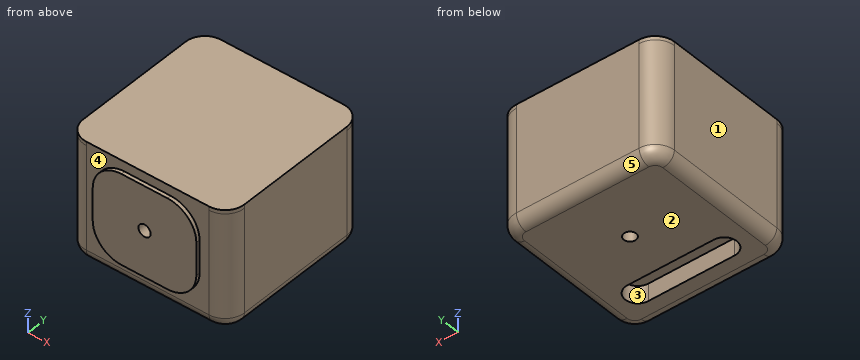
```python
from build123d import *

# Parameters (mm, degrees)
ESQUISSE1_W             = 84
ESQUISSE1_H             = 84
BOSS_EXTRU_1_DEPTH      = 60
CONG_1_R                = 10
CONG_2_R                = 6
BOSS_EXTRU_2_DEPTH      = 2
ESQUISSE5_R             = 3.175
ENL_V_MAT_EXTRU_1_DEPTH = 6
ENL_V_MAT_EXTRU_2_DEPTH = 9
ESQUISSE7_R             = 3.175
ENL_V_MAT_EXTRU_3_DEPTH = 6
BOSS_EXTRU_3_START      = 2
BOSS_EXTRU_3_DEPTH      = 2


with BuildPart() as part:
    # Esquisse1 → Boss.-Extru.1 (new body)
    with BuildSketch(Plane.XY):
        with Locations((12.35180193, 14.109375)):
            Rectangle(ESQUISSE1_W, ESQUISSE1_H)
    extrude(amount=BOSS_EXTRU_1_DEPTH)

    # Congé1
    cong_1_edges = [part.edges().sort_by_distance(p)[0] for p in [
        (-29.64819807, 56.109375, 30),
        (54.35180193, 56.109375, 30),
        (54.35180193, -27.890625, 30),
        (-29.64819807, -27.890625, 30),
    ]]
    fillet(cong_1_edges, radius=CONG_1_R)

    # Congé2
    cong_2_edges = [part.edges().sort_by_distance(p)[0] for p in [
        (12.35180193, -27.890625, 0),
        (-29.64819807, 14.109375, 0),
        (12.35180193, 56.109375, 0),
        (54.35180193, 14.109375, 0),
        (51.422869741, 53.180442812, 0),
        (-26.719265882, 53.180442812, 0),
        (51.422869741, -24.961692812, 0),
        (-26.719265882, -24.961692812, 0),
    ]]
    fillet(cong_2_edges, radius=CONG_2_R)

    # Esquisse2 → Boss.-Extru.2 (add)
    with BuildSketch(Plane.XZ.offset(27.890625)):
        with BuildLine():
            Line((24.35180193, 57), (0.35180193, 57))
            ThreePointArc((0.35180193, 57), (-10.254799788, 52.606601718), (-14.64819807, 42))
            Line((-14.64819807, 42), (-14.64819807, 25))
            ThreePointArc((-14.64819807, 25), (-10.254799788, 14.393398282), (0.35180193, 10))
            Line((0.35180193, 10), (24.35180193, 10))
            ThreePointArc((24.35180193, 10), (34.958403647, 14.393398282), (39.35180193, 25))
            Line((39.35180193, 25), (39.35180193, 42))
            ThreePointArc((39.35180193, 42), (34.958403647, 52.606601718), (24.35180193, 57))
        make_face()
    extrude(amount=BOSS_EXTRU_2_DEPTH)

    # Esquisse5 → Enlèv. mat.-Extru.1 (cut)
    with BuildSketch(Plane.XZ.offset(29.890625)):
        with Locations(Location((12.35180193, 34, 0), (0, 0, 270))):
            Circle(ESQUISSE5_R)
    extrude(amount=-ENL_V_MAT_EXTRU_1_DEPTH, mode=Mode.SUBTRACT)

    # Esquisse6 → Enlèv. mat.-Extru.2 (cut)
    with BuildSketch(Plane(origin=(0, 0, 0), x_dir=(-1, 0, 0), z_dir=(0, 0, -1))):
        with BuildLine():
            Line((-34.85180193, -1.890625), (10.14819807, -1.890625))
            ThreePointArc((10.14819807, -1.890625), (16.64819807, -8.390625), (10.14819807, -14.890625))
            Line((10.14819807, -14.890625), (-34.85180193, -14.890625))
            ThreePointArc((-34.85180193, -14.890625), (-41.35180193, -8.390625), (-34.85180193, -1.890625))
        make_face()
    extrude(amount=-ENL_V_MAT_EXTRU_2_DEPTH, mode=Mode.SUBTRACT)

    # Esquisse7 → Enlèv. mat.-Extru.3 (cut)
    with BuildSketch(Plane(origin=(0, 0, 0), x_dir=(-1, 0, 0), z_dir=(0, 0, -1))):
        with Locations((-14.35180193, 21.109375)):
            Circle(ESQUISSE7_R)
    extrude(amount=-ENL_V_MAT_EXTRU_3_DEPTH, mode=Mode.SUBTRACT)

    # Esquisse8 → Boss.-Extru.3 (add)
    with BuildSketch(Plane.XY.offset(60).offset(BOSS_EXTRU_3_START)):
        with BuildLine():
            Line((-19.64819807, 56.109375), (44.35180193, 56.109375))
            ThreePointArc((44.35180193, 56.109375), (51.422869741, 53.180442812), (54.35180193, 46.109375))
            Line((54.35180193, 46.109375), (54.35180193, -17.890625))
            ThreePointArc((54.35180193, -17.890625), (51.422869741, -24.961692812), (44.35180193, -27.890625))
            Line((44.35180193, -27.890625), (-19.64819807, -27.890625))
            ThreePointArc((-19.64819807, -27.890625), (-26.719265882, -24.961692812), (-29.64819807, -17.890625))
            Line((-29.64819807, -17.890625), (-29.64819807, 46.109375))
            ThreePointArc((-29.64819807, 46.109375), (-26.719265882, 53.180442812), (-19.64819807, 56.109375))
        make_face()
    extrude(amount=-BOSS_EXTRU_3_DEPTH)


solid = part.part
```
CAD build for the part. Positions are in the model's coordinates, mm. Face numbers are marked on the shaded views. A direction names the side the tool comes from. Coordinates: 2 decimals unless noted, no trailing zeros. Order: outer loops, then holes, each group sorted by start corner. A loop starts at its lowest first (then second) coordinate and runs counter-clockwise, first axis right, second up. Notation, with made-up numbers: (52.25, 40) - (73.25, 40) arc R31 cw to (73.25, 67) - close; hole circle Ø1 at (44.25, 24). An arc over 180 degrees is marked (long way). Answer in a Markdown table with one row per item.
1. Pull direction X, two halves, no side cores. Call the marked faces 1, 2 and 3: +X half, -X half, draft (parallel to the pull), parting line (faces both ways), or undercut.
Answer:
| item | result |
|---|---|
| face 1 | -X half |
| face 2 | draft |
| face 3 | undercut |
2. Flat gauge pins, fed straight in: P1, Ø0.6, axis at y = -29, z = 29.5, coming from the +X side; P2, Ø5, axis at x = 12.35, z = 34, coming from the -Y side; P3, Ø10, axis at x = 13.5, z = 4, coming from the +Y side; P4, Ø1, axis at x = -20, z = 46, coming from the -Y side. Where does each tip first touch, or does it go through?
Answer:
| item | result |
|---|---|
| P1 | x = 39.35 |
| P2 | y = -23.89 |
| P3 | y = 56.11 |
| P4 | y = -27.89 |
3. Slice it at C-C, the plane z = 55. List the corners of the cut face in (x, y).
Answer:
| item | result |
|---|---|
| outline | (-29.65, -17.89) arc R10 ccw to (-19.65, -27.89) - (-7.13, -27.89) - (-7.13, -29.89) - (31.84, -29.89) - (31.84, -27.89) - (44.35, -27.89) arc R10 ccw to (54.35, -17.89) - (54.35, 46.11) arc R10 ccw to (44.35, 56.11) - (-19.65, 56.11) arc R10 ccw to (-29.65, 46.11) - close |
4. 3-axis set-ups, long thin cutter, end or side, ignore diameter. For the marked faces 4 and 5: which of +Z, -Z, +X, -X, +Y, -Y reach the whole face in a straight line?
Answer:
| item | result |
|---|---|
| face 4 | -Y |
| face 5 | -Z, +X, -X, +Y |
5. Drill centre lines: L1, parallel to X at y = -28.5, z = 34; L2, parallel to X at y = -18.5, z = 47.5; L3, parallel to Z at x = -7, y = 50.5. Where is each one in solid material? Low to high. Write a range as from..to.
Answer:
| item | result |
|---|---|
| L1 | -14.65..9.18, 15.53..39.35 |
| L2 | -29.63..54.33 |
| L3 | 0.01..62 |
6. Slice it at B-B, the plane x = 33.5. List the corners of the cut face in (y, z).
Answer:
| item | result |
|---|---|
| outline | (-29.89, 13.11) - (-27.89, 13.11) - (-27.89, 6) arc R6 ccw to (-21.89, 0) - (-14.89, 0) - (-14.89, 9) - (-1.89, 9) - (-1.89, 0) - (50.11, 0) arc R6 ccw to (56.11, 6) - (56.11, 62) - (-27.89, 62) - (-27.89, 53.89) - (-29.89, 53.89) - close |
7. Slice it at D-D, the plane x = 42.5. List the corners of the cut face in (y, z).
Answer:
| item | result |
|---|---|
| outline | (-27.89, 6) arc R6 ccw to (-21.89, 0) - (50.11, 0) arc R6 ccw to (56.11, 6) - (56.11, 62) - (-27.89, 62) - close |
8. Slice it at A-A, the plane z = 34. List the corners of the cut face in (x, y), then the cut area to 3 significant figures.
Answer:
| item | result |
|---|---|
| outline | (-29.65, -17.89) arc R10 ccw to (-19.65, -27.89) - (-14.65, -27.89) - (-14.65, -29.89) - (9.18, -29.89) - (9.18, -23.89) - (15.53, -23.89) - (15.53, -29.89) - (39.35, -29.89) - (39.35, -27.89) - (44.35, -27.89) arc R10 ccw to (54.35, -17.89) - (54.35, 46.11) arc R10 ccw to (44.35, 56.11) - (-19.65, 56.11) arc R10 ccw to (-29.65, 46.11) - close |
| area | 7,040 mm² |
